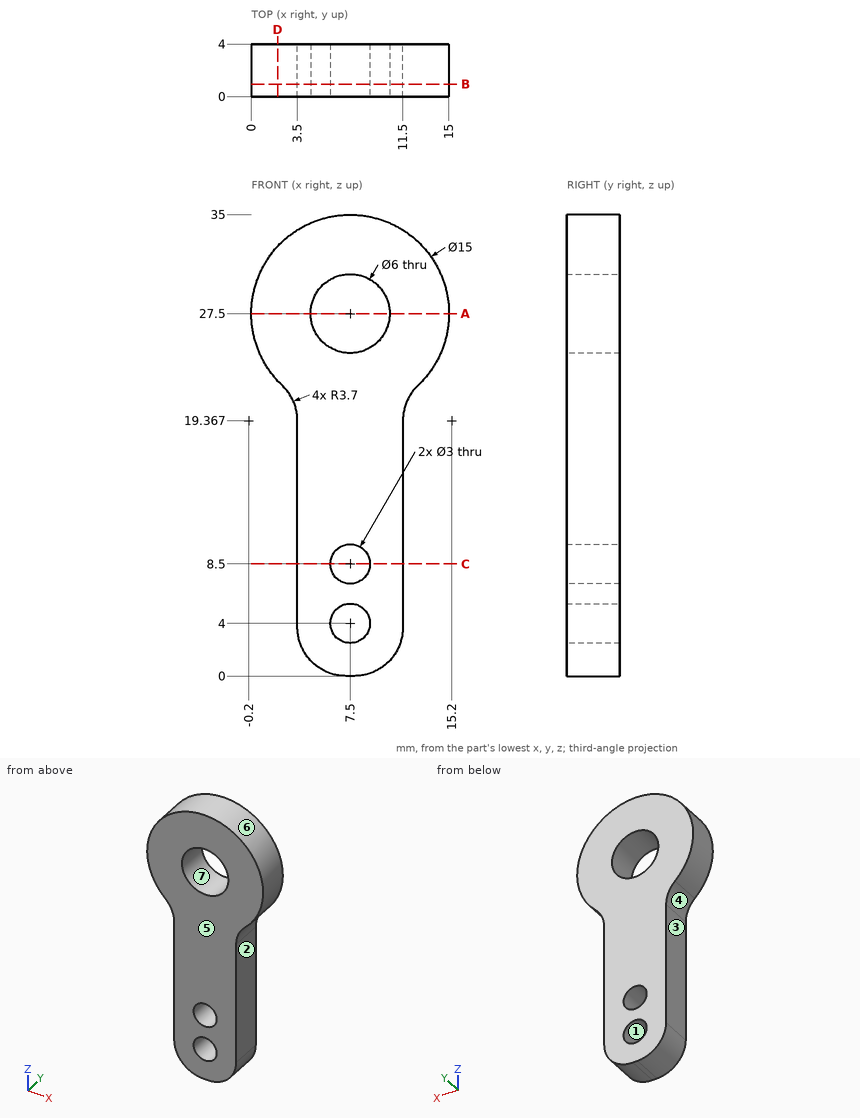
Geometry check sheet. Reference: drawing and pictorial views, mm from the part's lowest x, y, z. A direction names the side the tool comes from. Give positions to 0.01 mm unless a question says otherwise; leave off trailing zeros. Order: outer loops, then holes, each group sorted by start corner. A loop starts at its lowest first (then second) coordinate and runs counter-clockwise, first axis right, second up. Notation, with made-up numbers: (-14, 34) - (28, 34) arc R23 cw to (28, 60) - close; hole circle Ø2 at (40.25, 5). An arc over 180 degrees is marked (long way). Answer as CSV lines item,"result". Start each with the question number.
Item 1: Section check D-D, the plane x = 2. Record the boundary of the cut face in (y, z), plus the area to 3 significant figures.
Item 2: Mould release check, pull along X, two halves, no side actions. Record for the marked faces 4, 5, 6 and 7: released by +X, released by -X, zero draft, split by the parting line, or undercut.
Item 3: Gauge pin test, flat ends, axial feed: pin 1 (2 mm diameter, centred on y = 3, z = 17.5, fed in from -X); pin 2 (1.2 mm diameter, centred on y = 1.5, z = 13.5, fed in from +X); pin 3 (8 mm diameter, centred on x = 7, z = 9.5, fed in from +Y); pin 4 (1.8 mm diameter, centred on x = 7.5, z = 4, fed in from -Y) (1 decimal). Record the tip position at first contact, or that the pin passes through.
Item 4: Section check B-B, the plane y = 0.95. Record the boundary of the cut face in (x, z).
Item 5: Section check A-A, the plane z = 27.5. Record the boundary of the cut face in (x, y).
Item 6: Section check C-C, the plane z = 8.5. Record the boundary of the cut face in (x, y), plus the area to 3 significant figures.
Item 7: Material ranges on L1, parallel to X at y = 2.6, z = 4; L2, parallel to X at y = 1.9, z = 27.5; L3, parallel to X at y = 0.9, z = 14.5, recorded low to high.
Item 8: Access from +Z, -Z, +X, -X, +Y, -Y to the whole of each face (thin tool, end or side, straight path). Record for the marked faces 1, 2 and 3.
Filled in:
1,outline,"(0, 22.4) - (4, 22.4) - (4, 32.6) - (0, 32.6) - close"
1,area,"40.8 mm^2"
2,face 4,"released by -X"
2,face 5,"zero draft"
2,face 6,"split by the parting line"
2,face 7,"undercut"
3,pin 1,"x = 3.5"
3,pin 2,"x = 11.5"
3,pin 3,"y = 4"
3,pin 4,"through"
4,outline,"(2.34, 22.05) arc R3.7 cw to (3.5, 19.37) - (3.5, 3.7) arc R3.7 ccw to (7.2, 0) - (7.8, 0) arc R3.7 ccw to (11.5, 3.7) - (11.5, 19.37) arc R3.7 cw to (12.66, 22.05) arc R7.5 ccw (long way) to start; hole circle Ø6 at (7.5, 27.5); hole circle Ø3 at (7.5, 4); hole circle Ø3 at (7.5, 8.5)"
5,outline,"(0, 0) - (4.5, 0) - (4.5, 4) - (0, 4) - close; (10.5, 0) - (15, 0) - (15, 4) - (10.5, 4) - close"
6,outline,"(3.5, 0) - (6, 0) - (6, 4) - (3.5, 4) - close; (9, 0) - (11.5, 0) - (11.5, 4) - (9, 4) - close"
6,area,"20.0 mm^2"
7,L1,"3.5 to 6, 9 to 11.5"
7,L2,"0 to 4.5, 10.5 to 15"
7,L3,"3.5 to 11.5"
8,face 1,"+Y, -Y"
8,face 2,"-Z, +X, +Y, -Y"
8,face 3,"-Z, -X, +Y, -Y"
